from build123d import *

# Parameters (mm, degrees)
SKETCH1_W           = 78
SKETCH1_H           = 63
SKETCH1_R           = 8
SKETCH1_R_2         = 4
SKETCH1_W_2         = 27
SKETCH1_H_2         = 15
BOSS_EXTRUDE1_DEPTH = 2


with BuildPart() as part:
    # Sketch1 → Boss-Extrude1 (new body)
    with BuildSketch(Plane.XY):
        Rectangle(SKETCH1_W, SKETCH1_H)
        with Locations(Location((23, 15.5, 0), (0, 0, 180))):
            Circle(SKETCH1_R, mode=Mode.SUBTRACT)
        with Locations((0, 15.5)):
            Circle(SKETCH1_R_2, mode=Mode.SUBTRACT)
        with Locations((-23, -17.5)):
            Circle(SKETCH1_R_2, mode=Mode.SUBTRACT)
        with Locations(Location((23, -2.5, 0), (0, 0, 180))):
            Circle(SKETCH1_R_2, mode=Mode.SUBTRACT)
        with Locations(Location((23, -17.5, 0), (0, 0, 180))):
            Circle(SKETCH1_R_2, mode=Mode.SUBTRACT)
        with Locations((-23, -2.5)):
            Circle(SKETCH1_R_2, mode=Mode.SUBTRACT)
        with Locations((-23, 15.5)):
            Circle(SKETCH1_R, mode=Mode.SUBTRACT)
        with Locations((0, -8)):
            Rectangle(SKETCH1_W_2, SKETCH1_H_2, mode=Mode.SUBTRACT)
    extrude(amount=BOSS_EXTRUDE1_DEPTH)


solid = part.part
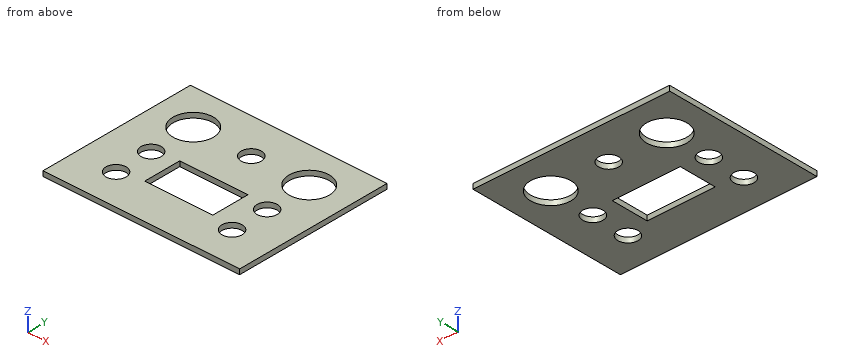
Here's how the part is built. I have some questions about the finished solid (model axes, mm). Coordinates: 2 decimals unless noted, no trailing zeros. Order: outer loops, then holes, each group sorted by start corner. A loop starts at its lowest first (then second) coordinate and runs counter-clockwise, first axis right, second up. Notation, with made-up numbers: M 0,74.25 L 35,74.25 A25 ccw 35,108.25 Z; hole C 14.25,27.5 d11. An arc over 180 degrees is marked long. Answer as CSV lines item,"result".
Item 1: Imagine slicing it at D-D on x = 16. Write out the boundary of the cut face in (y, z).
Results found:
outline,"M -31.5,0 L 11.63,0 L 11.63,2 L -31.5,2 Z; M 19.37,0 L 31.5,0 L 31.5,2 L 19.37,2 Z"
Item 2: Imagine slicing it at A-A on z = 1.4. Give the number of separate pieces and of enclosed holes in the cut face, plus the area to 3 significant figures.
Results found:
separate pieces,"1"
enclosed holes,"8"
area,"3,860 mm2"
Item 3: Imagine slicing it at B-B on y = -2.5. Write out the boundary of the cut face in (x, z), plus the area to 3 significant figures.
Results found:
outline,"M -39,0 L -27,0 L -27,2 L -39,2 Z; M -19,0 L -13.5,0 L -13.5,2 L -19,2 Z; M 13.5,0 L 19,0 L 19,2 L 13.5,2 Z; M 27,0 L 39,0 L 39,2 L 27,2 Z"
area,"70.0 mm2"
Item 4: If I drill on line 1 (Y direction, x = 23, z = 1.55); line 2 (Y direction, x = 0, z = 0.95); line 3 (Y direction, x = -26, z = 0.2), over which ranges is the centre line in solid material (lowest first)?
Results found:
line 1,"-31.5 to -21.5, -13.5 to -6.5, 1.5 to 7.5, 23.5 to 31.5"
line 2,"-31.5 to -15.5, -0.5 to 11.5, 19.5 to 31.5"
line 3,"-31.5 to -20.15, -14.85 to -5.15, 0.15 to 8.08, 22.92 to 31.5"
Item 5: Imagine slicing it at C-C on x = 0. Write out the boundary of the cut face in (y, z), plus the area to 3 significant figures.
Results found:
outline,"M -31.5,0 L -15.5,0 L -15.5,2 L -31.5,2 Z; M -0.5,0 L 11.5,0 L 11.5,2 L -0.5,2 Z; M 19.5,0 L 31.5,0 L 31.5,2 L 19.5,2 Z"
area,"80.0 mm2"
